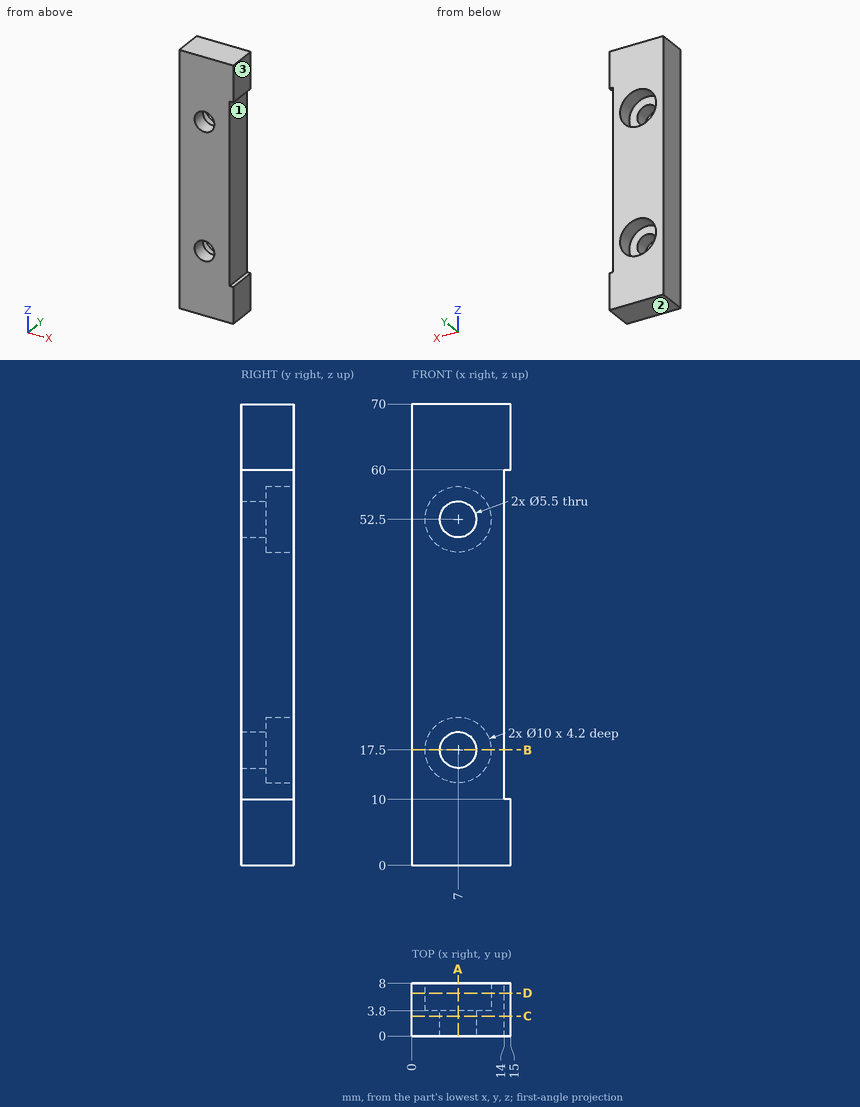
Geometry check sheet. Reference: drawing and pictorial views, mm from the part's lowest x, y, z. Coordinates: 2 decimals unless noted, no trailing zeros. Order: outer loops, then holes, each group sorted by start corner. A loop starts at its lowest first (then second) coordinate and runs counter-clockwise, first axis right, second up.
Item 1: Scan lines: line 1 along Z through (x, y) = (6.75, 0.5); line 2 along Z through (x, y) = (7, 6.5); line 3 along X through (y, z) = (2.4, 17.5). Record each from-to range of solid material in increasing order.
Item 2: Mould release check, pull along Z, two halves, no side actions. Record for the marked faces 1, 2 and 3: released by +Z, released by -Z, zero draft, split by the parting line, or undercut.
Item 3: Section check B-B (z = 17.5). Enter the section's corners in (x, y), plus the area to 3 significant figures.
Item 4: Section check D-D (y = 6.5). Enter the section's corners in (x, z), plus the area to 3 significant figures.
Item 5: Depth check by flat-ended pin: pin 1 (5 mm diameter, centred on x = 7, z = 52.5, fed in from +Y); pin 2 (8 mm diameter, centred on x = 7, z = 52.5, fed in from +Y); pin 3 (2.5 mm diameter, centred on y = 3.5, z = 40, fed in from +X). Enter the tip coordinate at first touch or a pass-through.
Item 6: Section check C-C (y = 3). Enter the section's corners in (x, z).
Item 7: Section check A-A (x = 7). Enter the section's corners in (y, z).
Check sheet entries:
1. line 1: z = 0 to 14.76, 20.24 to 49.76, 55.24 to 70
1. line 2: z = 0 to 12.5, 22.5 to 47.5, 57.5 to 70
1. line 3: x = 0 to 4.25, 9.75 to 14
2. face 1: undercut
2. face 2: released by -Z
2. face 3: zero draft
3. outline: (0, 0) - (4.25, 0) - (4.25, 3.8) - (2, 3.8) - (2, 8) - (0, 8) - close; (9.75, 0) - (14, 0) - (14, 8) - (12, 8) - (12, 3.8) - (9.75, 3.8) - close
3. area: 49.1 mm2
4. outline: (0, 0) - (15, 0) - (15, 10) - (14, 10) - (14, 60) - (15, 60) - (15, 70) - (0, 70) - close; hole circle Ø10 at (7, 17.5); hole circle Ø10 at (7, 52.5)
4. area: 843 mm2
5. pin 1: passes through
5. pin 2: stops at y = 3.8
5. pin 3: stops at x = 14
6. outline: (0, 0) - (15, 0) - (15, 10) - (14, 10) - (14, 60) - (15, 60) - (15, 70) - (0, 70) - close; hole circle Ø5.5 at (7, 17.5); hole circle Ø5.5 at (7, 52.5)
7. outline: (0, 0) - (8, 0) - (8, 12.5) - (3.8, 12.5) - (3.8, 14.75) - (0, 14.75) - close; (0, 20.25) - (3.8, 20.25) - (3.8, 22.5) - (8, 22.5) - (8, 47.5) - (3.8, 47.5) - (3.8, 49.75) - (0, 49.75) - close; (0, 55.25) - (3.8, 55.25) - (3.8, 57.5) - (8, 57.5) - (8, 70) - (0, 70) - close
